from build123d import *

# Parameters (mm, degrees)
SKETCH1_W           = 20
SKETCH1_H           = 20
SKETCH1_W_2         = 17.1
SKETCH1_H_2         = 17.1
BOSS_EXTRUDE1_DEPTH = 194
SKETCH2_R           = 2.05
CUT_EXTRUDE1_DEPTH  = 21


with BuildPart() as part:
    # Sketch1 → Boss-Extrude1 (new body)
    with BuildSketch(Plane(origin=(0, 0, 0), x_dir=(1, 0, 0), z_dir=(0, 1, 0))):
        with Locations((10, 10)):
            Rectangle(SKETCH1_W, SKETCH1_H)
        with Locations((10, 10)):
            Rectangle(SKETCH1_W_2, SKETCH1_H_2, mode=Mode.SUBTRACT)
    extrude(amount=BOSS_EXTRUDE1_DEPTH)

    # Sketch2 → Cut-Extrude1 (cut, through all)
    with BuildSketch(Plane.ZY):
        with Locations((-10, 187)):
            Circle(SKETCH2_R)
        with Locations((-10, 157)):
            Circle(SKETCH2_R)
        with Locations((-10, 37)):
            Circle(SKETCH2_R)
        with Locations((-10, 7)):
            Circle(SKETCH2_R)
    extrude(amount=-CUT_EXTRUDE1_DEPTH, mode=Mode.SUBTRACT)


solid = part.part
Input: part model. Units: mm. Frame: model coordinates. A direction names the side the tool comes from. Round coordinates to 2 decimals unless told otherwise and drop trailing zeros. Loops run counter-clockwise (first coordinate to the right, second up) from the corner with the lowest first, then second, coordinate; pieces in that order, holes last. Notation, with made-up numbers: (-35.5, 59) -> (19.5, 59) arc R33 cw to (19.5, 96) -> close; hole circle Ø8 at (74.25, -30). An arc over 180 degrees is marked (long way). Answer as a JSON object with one key per item and string values. Group by question number.
1) Ray query, L1, parallel to Y at x = 19.6, z = -10; L2, parallel to X at y = 154, z = -18.25; L3, parallel to Z at x = 16.75, y = 140. Return the intervals inside material, ascending.
2) Draft query along X for faces 1 (the flat face through (10, 96, -1.45)), 2 (the flat face through (20, 96, -10)), 3 (the flat face through (1.45, 96, -10)), 4 (the flat face through (10, 96, 0)). Return one class per face: +X half, -X half, draft (parallel to the pull), parting line (faces both ways), or undercut.
3) Section query D-D on y = 163. Output: boundary loops of the cut face in (x, z).
4) Reachability of faces 5 (the cylindrical face through (0.715, 39.033, -10.267)), 6 (the flat face through (10, 96, -18.55)) from +Z, -Z, +X, -X, +Y, -Y: full face, straight path, thin tool, end or side. Return the list, or none.
5) Section query A-A on z = -14.5. Output: boundary loops of the cut face in (x, y).
6) Section query C-C on y = 37. Output: boundary loops of the cut face in (x, z), plus the area to 3 significant figures.
7) Pin query (flat end, axial travel): pin 1 (2.5 mm diameter, centred on y = 7, z = -10, fed in from -X). Return the tip coordinate at first contact, or that it passes through.
8) Section query B-B on x = 9.5. Output: boundary loops of the cut face in (y, z), plus the area to 3 significant figures.
Reply:
{
 "1": {"L1": "y = 0 to 4.95, 9.05 to 34.95, 39.05 to 154.95, 159.05 to 184.95, 189.05 to 194", "L2": "x = 0 to 1.45, 18.55 to 20", "L3": "z = -20 to -18.55, -1.45 to 0"},
 "2": {"face 1": "undercut", "face 2": "+X half", "face 3": "undercut", "face 4": "draft"},
 "3": {"outline": "(0, -20) -> (20, -20) -> (20, 0) -> (0, 0) -> close; hole (1.45, -18.55) -> (18.55, -18.55) -> (18.55, -1.45) -> (1.45, -1.45) -> close"},
 "4": {"face 5": "+X, -X", "face 6": "+Y, -Y"},
 "5": {"outline": "(0, 0) -> (1.45, 0) -> (1.45, 194) -> (0, 194) -> close; (18.55, 0) -> (20, 0) -> (20, 194) -> (18.55, 194) -> close"},
 "6": {"outline": "(0, -20) -> (20, -20) -> (20, -12.05) -> (18.55, -12.05) -> (18.55, -18.55) -> (1.45, -18.55) -> (1.45, -12.05) -> (0, -12.05) -> close; (0, -7.95) -> (1.45, -7.95) -> (1.45, -1.45) -> (18.55, -1.45) -> (18.55, -7.95) -> (20, -7.95) -> (20, 0) -> (0, 0) -> close", "area": "95.7 mm2"},
 "7": {"pin 1": "passes through"},
 "8": {"outline": "(0, -20) -> (194, -20) -> (194, -18.55) -> (0, -18.55) -> close; (0, -1.45) -> (194, -1.45) -> (194, 0) -> (0, 0) -> close", "area": "563 mm2"}
}
